For this review, take the finished solid that the model builds, in its own axes (mm). Face numbers are marked on the shaded views. Round coordinates to 2 decimals unless told otherwise and drop trailing zeros. Order: outer loops, then holes, each group sorted by start corner. A loop starts at its lowest first (then second) coordinate and runs counter-clockwise, first axis right, second up. Notation, with made-up numbers: M -8,-13.5 L 6,-13.5 A28 ccw 6,17.5 Z; hole C 65.25,63 d3. An arc over 180 degrees is marked long. Answer as a JSON object with one key per item and string values.
from build123d import *

# Parameters (mm, degrees)
F0_R     = 1.25
F1_DEPTH = 12
F2_DEPTH = 12
F3_SIZE  = 0.15


with BuildPart() as f1:
    # F0 (on Top) → F1 (new body)
    with BuildSketch(Plane.XY):
        Polygon((1.433978, -2.505426), (2.886751, -0.010851), (1.452773, 2.494574), (-1.433978, 2.505426), (-2.886751, 0.010851), (-1.452773, -2.494574), align=None)
        Circle(F0_R, mode=Mode.SUBTRACT)
    extrude(amount=F1_DEPTH)

    # F0 (on Top) → F2 (cut)
    with BuildSketch(Plane.XY):
        Polygon((1.433978, -2.505426), (2.886751, -0.010851), (1.452773, 2.494574), (-1.433978, 2.505426), (-2.886751, 0.010851), (-1.452773, -2.494574), align=None)
        Circle(F0_R, mode=Mode.SUBTRACT)
    extrude(amount=-F2_DEPTH, mode=Mode.SUBTRACT)

    # F3
    f3_edges = [f1.edges().sort_by_distance(p)[0] for p in [
        (1.25, 0, 6),
        (-1.25, 0, 0),
        (-1.25, 0, 12),
    ]]
    chamfer(f3_edges, length=F3_SIZE)


solid = f1.part
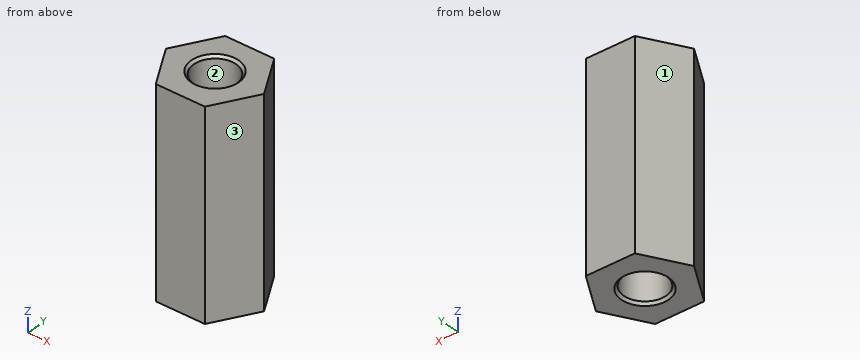
1) Insertion check: P1, Ø2, axis at x = 0, y = 0, coming from the +Z side. The pin has a flat end and moves straight along its axis. Give the tip position at first contact, or say it passes through.
Geometry check:
{"P1": "passes through"}
2) Add section A-A on x = 0. State the section outline as (y, z) points, and give its area (3 significant figures).
Geometry check:
{"outline": "M -2.5,0 L -1.4,0 L -1.25,0.15 L -1.25,11.85 L -1.4,12 L -2.5,12 Z; M 1.25,0.15 L 1.4,0 L 2.5,0 L 2.5,12 L 1.4,12 L 1.25,11.85 Z", "area": "30.0 mm²"}
3) Add section B-B on x = -2.2. State the section outline as (y, z) points.
Geometry check:
{"outline": "M -1.19,0 L 1.19,0 L 1.19,12 L -1.19,12 Z"}
4) For L1, parallel to Y at x = 0.3, z = 2.25; L2, parallel to X at y = -0.4, z = 8.75; L3, parallel to Y at x = 1, z = 7.5, list the stretches that pass through material, from the lowest coordinate up.
Geometry check:
{"L1": "y = -2.5 to -1.21, 1.21 to 2.5", "L2": "x = -2.65 to -1.18, 1.18 to 2.66", "L3": "y = -2.5 to -0.75, 0.75 to 2.5"}
5) Mouldability with a two-part tool opening along X and no side actions: class the marked faces 1, 2 and 3 as +X half, -X half, draft (parallel to the pull), parting line (faces both ways), or undercut.
Geometry check:
{"face 1": "-X half", "face 2": "undercut", "face 3": "+X half"}
